Here's how the part is built. I have some questions about the finished solid (model axes, mm). Face numbers are marked on the shaded views. A direction names the side the tool comes from. Coordinates: 2 decimals unless noted, no trailing zeros. Write each loop counter-clockwise with the first axis right and the second up, starting at its lowest first coordinate (ties: lowest second). Pieces come first, ordered by that corner, then holes. Notation, with made-up numbers: (-17.5, 81.25) -> (24.5, 81.25) arc R31 ccw to (24.5, 116.25) -> close; hole circle Ø4 at (76.5, 36). An arc over 180 degrees is marked (long way). Put each result on its own line as item: value.
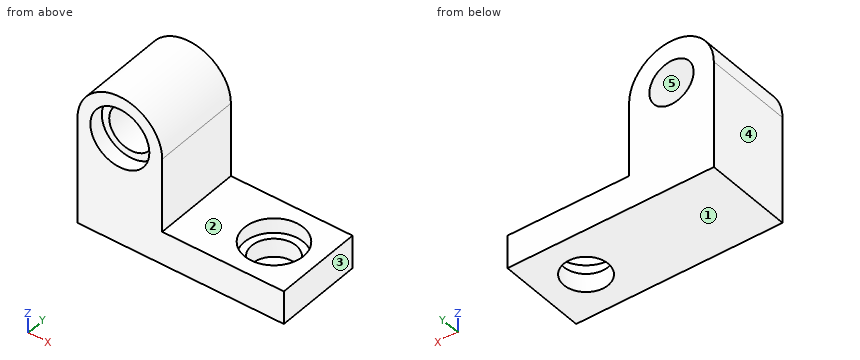
```python
from build123d import *

# Parameters (mm, degrees)
F0_W           = 125.521261
F0_H           = 76.2
F1_DEPTH       = 28.575
F3_D           = 38.1
F3_CBORE_D     = 50.8
F3_CBORE_DEPTH = 12.7
F5_DEPTH       = 76.2
F6_D           = 38.1
F6_CBORE_D     = 50.8
F6_CBORE_DEPTH = 12.7


with BuildPart() as f1:
    # F0 (on Top) → F1 (new body)
    with BuildSketch(Plane.XY):
        with Locations((26.139369, 0)):
            Rectangle(F0_W, F0_H)
    extrude(amount=F1_DEPTH)

    # F3 (through all)
    with Locations(Plane.XY.offset(28.575)):
        with Locations((50.8, 0)):
            CounterBoreHole(F3_D / 2, F3_CBORE_D / 2, F3_CBORE_DEPTH)

    # F4 (on face) → F5 (join)
    with BuildSketch(Plane.XZ.offset(38.1)):
        Polygon((-88.9, 92.346745), (-88.9, 0), (-36.621261, 0), (-36.621261, 28.575), (-15.875, 28.575), (-15.875, 92.346745), align=None)
        with BuildLine():
            ThreePointArc((-15.875, 92.346745), (-52.3875, 128.859245), (-88.9, 92.346745))
            Line((-88.9, 92.346745), (-15.875, 92.346745))
        make_face()
    extrude(amount=-F5_DEPTH)

    # F6 (through all)
    with Locations(Plane.XZ.offset(38.1)):
        with Locations((-52.3875, 92.346745)):
            CounterBoreHole(F6_D / 2, F6_CBORE_D / 2, F6_CBORE_DEPTH)


solid = f1.part
```
Item 1: Imagine slicing it at A-A on y = 0. State how many separate pieces and enclosed holes the cut face has, then the cut area to 3 significant figures.
Output:
separate pieces: 2
enclosed holes: 1
area: 9,440 mm²
Item 2: Imagine slicing it at C-C on y = -27.5. Write out the boundary of the cut face in (x, z) (1 decimal), then the cut area to 3 significant figures.
Output:
outline: (-88.9, 0) -> (88.9, 0) -> (88.9, 28.6) -> (-15.9, 28.6) -> (-15.9, 92.3) arc R36.5 ccw to (-88.9, 92.3) -> close; hole circle Ø50.8 at (-52.4, 92.3)
area: 9,800 mm²
Item 3: Which directions (+Z, -Z, +X, -X, +Y, -Y) give clear straight access to the entire face, cutting with the end or side of a thin tool? Please do the marked faces 1 and 2.
Output:
face 1: -Z, +X, -X, +Y, -Y
face 2: +Z, +X, +Y, -Y
Item 4: For P1, Ø8, axis at y = 26.5, z = 115, coming from the -X side; P2, Ø5, axis at y = 27.5, z = 114, coming from the -X side; P3, Ø12, axis at x = 19, y = 29.5, coming from the +Z side (3 decimals); P4, Ø2, axis at x = -61.5, y = -16, coming from the -Z side, each with a flat end and sliding along its axis, tell me the tip position at first contact or that it passes through.
Output:
P1: stops at x = -83.78
P2: stops at x = -83.47
P3: stops at z = 28.575
P4: stops at z = 0
Item 5: Imagine slicing it at D-D on z = 20. Write out the boundary of the cut face in (x, y).
Output:
outline: (-88.9, -38.1) -> (88.9, -38.1) -> (88.9, 38.1) -> (-88.9, 38.1) -> close; hole circle Ø50.8 at (50.8, 0)
Item 6: If we mould it in two halves opening along X, with no side actions, what happens to the marked faces 3, 4 and 5? For each: released by +X, released by -X, zero draft, split by the parting line, or undercut.
Output:
face 3: released by +X
face 4: released by -X
face 5: undercut
Item 7: Please list where these lines run through material, in increasing order: line 1 along Y through (x, z) = (50.8, 6.75); line 2 along X through (y, z) = (26.5, 46.5) (3 decimals); line 3 along Z through (x, y) = (68, -26.5) (3 decimals). Write a range as from..to.
Output:
line 1: y = -38.1..-19.05, 19.05..38.1
line 2: x = -88.9..-15.875
line 3: z = 0..28.575
Item 8: Imagine slicing it at B-B on x = 50.8. Write out the boundary of the cut face in (y, z) (3 decimals).
Output:
outline: (-38.1, 0) -> (-19.05, 0) -> (-19.05, 15.875) -> (-25.4, 15.875) -> (-25.4, 28.575) -> (-38.1, 28.575) -> close; (19.05, 0) -> (38.1, 0) -> (38.1, 28.575) -> (25.4, 28.575) -> (25.4, 15.875) -> (19.05, 15.875) -> close
